Can you work these out from the model? Positions are in its coordinate system, mm. A direction names the side the tool comes from. Coordinates: 2 decimals unless noted, no trailing zeros. Loops run counter-clockwise (first coordinate to the right, second up) from the corner with the lowest first, then second, coordinate; pieces in that order, holes last. Notation, with made-up numbers: (54.25, 0.5) -> (79.25, 0.5) arc R26 ccw to (79.25, 16.5) -> close; hole circle Ø2 at (5, -29.5). An arc over 180 degrees is marked (long way). Put each result on its own line as item: value. Start each with the question number.
Item 1: Will these pins go through, and if not, where does the flat tip stop? P1, Ø1.5, axis at y = 2, z = -13.5, coming from the -X side; P2, Ø1, axis at x = -5, y = 2.5, coming from the -Z side; P3, Ø1.5, axis at x = 20, y = 1.5, coming from the -Z side.
Item 2: We'd pull the mould along Z, two halves only. Please class faces 1 (the flat face through (20.824, 1.479, -7.06)), 2 (the flat face through (42.454, 1.521, -16.934)), 3 (the flat face through (22.61, 1.479, -13.344)): pulls with the +Z half, pulls with the -Z half, needs draft (parallel to the pull), parting line crosses it, or undercut.
Item 3: Please list where these lines run through material, in increasing order: L1, parallel to X at y = 2.4, z = -0.25; L2, parallel to X at y = 1.05, z = 1; L3, parallel to Z at x = -4, y = 1.8. Write a range as from..to.
Item 4: If we section it at D-D on z = -8: Please give me the cut outline in (x, y), plus the area to 3 significant figures.
Item 5: If we section it at C-C on x = 0.5: Please give me the cut outline in (y, z).
Item 6: For faces 4 (the flat face through (31.5, 1.5, -12.7)), 5 (the flat face through (0, 1, -5)), 6 (the cylindrical face through (-16, 1, 0)), which set-ups out of +Z, -Z, +X, -X, +Y, -Y let a thin tool reach every point of the face, with its end or its side?
Item 7: If we section it at B-B on z = 0: Please give me the cut outline in (x, y), plus the area to 3 significant figures.
Item 8: If we section it at A-A on y = 1.6: Please give me the cut outline in (x, z), plus the area to 3 significant figures.
```python
from build123d import *

# Parameters (mm, degrees)
IZIM2_R                     = 1.5
Y_KSEKLIK_EKSTR_ZYON1_DEPTH = 3
Y_KSEKLIK_EKSTR_ZYON2_START = -3
Y_KSEKLIK_EKSTR_ZYON2_DEPTH = 3
KES_EKSTR_ZYON1_DEPTH       = 3
KES_EKSTR_ZYON2_DEPTH       = 3
KES_EKSTR_ZYON3_DEPTH       = 3


with BuildPart() as part:
    # Çizim2 → Yükseklik-Ekstrüzyon1 (new body)
    with BuildSketch(Plane(origin=(0, 0, 0), x_dir=(1, 0, 0), z_dir=(0, 1, 0))):
        with BuildLine():
            Line((-11, 5), (11, 5))
            ThreePointArc((11, 5), (16, 0), (11, -5))
            Line((11, -5), (-11, -5))
            ThreePointArc((-11, -5), (-16, 0), (-11, 5))
        make_face()
        with Locations(Location((-11, 0, 0), (0, 0, 270))):
            Circle(IZIM2_R, mode=Mode.SUBTRACT)
        with Locations(Location((11, 0, 0), (0, 0, 270))):
            Circle(IZIM2_R, mode=Mode.SUBTRACT)
    extrude(amount=Y_KSEKLIK_EKSTR_ZYON1_DEPTH)

    # Çizim3 → Yükseklik-Ekstrüzyon2 (add)
    with BuildSketch(Plane(origin=(0, 3, 0), x_dir=(1, 0, 0), z_dir=(0, 1, 0)).offset(Y_KSEKLIK_EKSTR_ZYON2_START)):
        with BuildLine():
            Line((11, 5), (40.233453571, 26.009645221))
            Line((40.233453571, 26.009645221), (46.069466132, 17.889241451))
            Line((46.069466132, 17.889241451), (37.949062363, 12.05322889))
            Line((37.949062363, 12.05322889), (36.369445688, 14.251155139))
            Line((36.369445688, 14.251155139), (26.428767162, 11.088423867))
            Line((26.428767162, 11.088423867), (15.060201885, 2.918006281))
            ThreePointArc((15.060201885, 2.918006281), (13.281443468, 4.449158988), (11, 5))
        make_face()
    extrude(amount=Y_KSEKLIK_EKSTR_ZYON2_DEPTH)

    # Çizim4 → Kes-Ekstrüzyon1 (cut)
    with BuildSketch(Plane(origin=(0, 3, 0), x_dir=(1, 0, 0), z_dir=(0, 1, 0))):
        Polygon((34.549170932, 21.924436428), (40.233453571, 26.009645221), (42.567858595, 22.761483713), align=None)
    extrude(amount=-KES_EKSTR_ZYON1_DEPTH, mode=Mode.SUBTRACT)

    # Çizim5 → Kes-Ekstrüzyon2 (cut)
    with BuildSketch(Plane(origin=(0, 3, 0), x_dir=(1, 0, 0), z_dir=(0, 1, 0))):
        Polygon((38.76110274, 12.636830146), (36.369445688, 14.251155139), (37.949062363, 12.05322889), align=None)
        Polygon((37.993526442, 15.418357651), (38.76110274, 12.636830146), (40.385183494, 13.804032658), align=None)
        Polygon((39.617607196, 16.585560164), (40.385183494, 13.804032658), (42.009264247, 14.971235171), align=None)
        Polygon((41.24168795, 17.752762676), (42.009264247, 14.971235171), (43.633345001, 16.138437683), align=None)
        Polygon((42.865768704, 18.919965188), (43.633345001, 16.138437683), (45.257425755, 17.305640195), align=None)
        Polygon((44.489849458, 20.0871677), (45.257425755, 17.305640195), (46.069466132, 17.889241451), align=None)
    extrude(amount=-KES_EKSTR_ZYON2_DEPTH, mode=Mode.SUBTRACT)

    # Çizim6 → Kes-Ekstrüzyon3 (cut)
    with BuildSketch(Plane(origin=(0, 3, 0), x_dir=(1, 0, 0), z_dir=(0, 1, 0))):
        Polygon((15.060201885, 2.918006281), (14.736771564, -2.041177089), (11, -5), (11, -9.807776343), (27.690155634, -9.807776343), (28.885017057, 0.673945989), align=None)
    extrude(amount=-KES_EKSTR_ZYON3_DEPTH, mode=Mode.SUBTRACT)


solid = part.part
```
Solutions:
1. P1: x = 21.78
1. P2: z = -5
1. P3: z = -12.01
2. face 1: pulls with the +Z half
2. face 2: undercut
2. face 3: pulls with the -Z half
3. L1: -15.99..-12.48, -9.52..9.52, 12.48..14.89
3. L2: -15.9..-12.12, -9.88..9.88, 12.12..14.8
3. L3: -5..5
4. outline: (15.17, 0) -> (22.13, 0) -> (22.13, 3) -> (15.17, 3) -> close
4. area: 20.9 mm^2
5. outline: (0, -5) -> (3, -5) -> (3, 5) -> (0, 5) -> close
6. face 4: +Z, +Y, -Y
6. face 5: -Z, -X, +Y, -Y
6. face 6: -X, +Y, -Y
7. outline: (-16, 0) -> (-12.5, 0) -> (-12.5, 3) -> (-16, 3) -> close; (-9.5, 0) -> (9.5, 0) -> (9.5, 3) -> (-9.5, 3) -> close; (12.5, 0) -> (14.87, 0) -> (14.87, 3) -> (12.5, 3) -> close
7. area: 74.6 mm^2
8. outline: (-11, -5) -> (11, -5) -> (34.55, -21.92) -> (42.57, -22.76) -> (44.49, -20.09) -> (45.26, -17.31) -> (42.87, -18.92) -> (43.63, -16.14) -> (41.24, -17.75) -> (42.01, -14.97) -> (39.62, -16.59) -> (40.39, -13.8) -> (37.99, -15.42) -> (38.76, -12.64) -> (36.37, -14.25) -> (26.43, -11.09) -> (15.06, -2.92) -> (14.74, 2.04) -> (11, 5) -> (-11, 5) arc R5 ccw to start; hole circle Ø3 at (-11, 0); hole circle Ø3 at (11, 0)
8. area: 464 mm^2
